```python
from build123d import *

# Parameters (mm, degrees)
CONG_1_R           = 1
ESQUISSE2_W        = 30
ESQUISSE2_H        = 35
BOSS_EXTRU_1_DEPTH = 1


with BuildPart() as part:
    # Esquisse1 → Révolution1 (revolve)
    with BuildSketch(Plane.XY, mode=Mode.PRIVATE) as r_volution1_sk:
        Polygon((0, 19.136127235), (3, 19.136127235), (6.5, 23.136127235), (8.75, 23.136127235), (10, 4.136127235), (0, 4.136127235), align=None)
    revolve(r_volution1_sk.sketch.rotate(Axis((0, 0, 0), (0, 1, 0)), 90), axis=Axis((0, 0, 0), (0, 1, 0)))

    # Congé1
    cong_1_edges = [part.edges().sort_by_distance(p)[0] for p in [
        (0, 23.136127235, 8.75),
        (0, 23.136127235, 6.5),
    ]]
    fillet(cong_1_edges, radius=CONG_1_R)

    # Esquisse2 → Boss.-Extru.1 (add)
    with BuildSketch(Plane.XZ.offset(-4.136127235)):
        Rectangle(ESQUISSE2_W, ESQUISSE2_H)
    extrude(amount=BOSS_EXTRU_1_DEPTH)


solid = part.part
```
Source: CAD feature listing. Evaluate the final solid. Frame: model axes, mm. A direction names the side the tool comes from. Round coordinates to 2 decimals unless told otherwise and drop trailing zeros. Order: outer loops, then holes, each group sorted by start corner. A loop starts at its lowest first (then second) coordinate and runs counter-clockwise, first axis right, second up. Notation, with made-up numbers: (24.25, -1) -> (81.25, -1) arc R32 ccw to (81.25, 30) -> close; hole circle Ø7 at (47, 62). An arc over 180 degrees is marked (long way). One line per item, written item: value. Start each with the question number.
Q1. Section query D-D (y = 9). Return the cut outline in (x, z).
Q2. Section query C-C (y = 21.5). Return the cut outline in (x, z).
Q3. Section query B-B (z = 0). Return the cut outline in (x, y), plus the area to 3 significant figures.
Q4. Access query for faces 1 (the flat face through (-10.2, 4.136, 0.2)), 2 (the flat face through (-0.2, 3.6, 17.5)). Directions: +Z, -Z, +X, -X, +Y, -Y. A direction counts if a zero-diameter tool reaches every point of the face in a straight line with its end or side. Return the directions, or none.
Q5. Section query A-A (x = 0). Return the cut outline in (y, z), plus the area to 3 significant figures.
Q6. Draft query along Z for faces 3 (the flat face through (0, 19.136, 0)), 4 (the conical face through (3.12, 19.36, 0.69)), 5 (the flat face through (-0.2, 3.6, -17.5)), 6 (the flat face through (0, 3.136, 0)). Return one class per face: pulls with the +Z half, pulls with the -Z half, needs draft (parallel to the pull), parting line crosses it, or undercut.
Q7. Material intervals for probe 1 along Y at (x, z) = (-10.75, -13); probe 2 along X at (y, z) = (20.25, 1); probe 3 along X at (y, z) = (19.5, 4), sorted ascending.
Q8. Pin query (flat end, axial travel): pin 1 (3 mm diameter, centred on y = 18, z = -4.5, fed in from -X); pin 2 (12 mm diameter, centred on x = -10, z = 10, fed in from +Y); pin 3 (3 mm diameter, centred on x = -1.5, y = 15, fed in from +Z). Return the tip coordinate at first contact, or that it passes through.
Findings below:
1. outline: circle Ø19.36 at (0, 0)
2. outline: circle Ø17.72 at (0, 0); hole circle Ø10.14 at (0, 0)
3. outline: (-15, 3.14) -> (15, 3.14) -> (15, 4.14) -> (10, 4.14) -> (8.81, 22.2) arc R1 ccw to (7.81, 23.14) -> (6.95, 23.14) arc R1 ccw to (6.2, 22.79) -> (3, 19.14) -> (-3, 19.14) -> (-6.2, 22.79) arc R1 ccw to (-6.95, 23.14) -> (-7.81, 23.14) arc R1 ccw to (-8.81, 22.2) -> (-10, 4.14) -> (-15, 4.14) -> close
3. area: 348 mm²
4. face 1: +Y
4. face 2: +Z, +X, -X, +Y, -Y
5. outline: (3.14, -17.5) -> (4.14, -17.5) -> (4.14, -10) -> (22.2, -8.81) arc R1 ccw to (23.14, -7.81) -> (23.14, -6.95) arc R1 ccw to (22.79, -6.2) -> (19.14, -3) -> (19.14, 3) -> (22.79, 6.2) arc R1 ccw to (23.14, 6.95) -> (23.14, 7.81) arc R1 ccw to (22.2, 8.81) -> (4.14, 10) -> (4.14, 17.5) -> (3.14, 17.5) -> close
5. area: 353 mm²
6. face 3: undercut
6. face 4: undercut
6. face 5: pulls with the -Z half
6. face 6: needs draft
7. probe 1: 3.14 to 4.14
7. probe 2: -8.88 to -3.85, 3.85 to 8.88
7. probe 3: -8.05 to 8.05
8. pin 1: x = -8.59
8. pin 2: y = 23.08
8. pin 3: z = 9.35
